Read the model definition and answer for the solid it produces. Units are mm, in the model's axes. A direction names the side the tool comes from. Coordinates: 2 decimals unless noted, no trailing zeros. Order: outer loops, then holes, each group sorted by start corner. A loop starts at its lowest first (then second) coordinate and runs counter-clockwise, first axis right, second up. Notation, with made-up numbers: (46, -19) - (102, -19) arc R25 ccw to (102, 2) - close; hole circle Ø4 at (73.25, -4.75). An arc over 180 degrees is marked (long way). Write item = value, one per line.
Autodesk Fusion 360 part; units mm, degrees
sketch "Sketch1" plane through (0, 0, 0) normal (1, 0, 0) x (0, 1, 0) in component "Doorknob_Revolve_Addition"
  line L0 (0, 0) -> (0, 31.75)
  line L1 (-25.4, 3.175) -> (-25.4, 16.51)
  line L2 (-31.75, 16.51) -> (-31.75, 27.94)
  line L3 (-31.75, 27.94) -> (-38.1, 27.94)
  line L4 (-38.1, 27.94) -> (-38.1, 39.37)
  line L5 (-25.4, 16.51) -> (-31.75, 16.51)
  line L6 (-38.1, 39.37) -> (-44.45, 39.37)
  line L7 (-44.45, 39.37) -> (-44.45, 50.8)
  line L8 (-44.45, 50.8) -> (-50.8, 50.8)
  line L9 (-50.8, 50.8) -> (-50.8, 39.37)
  line L10 (-50.8, 39.37) -> (-57.15, 39.37)
  line L11 (-57.15, 39.37) -> (-57.15, 27.94)
  line L12 (-57.15, 27.94) -> (-63.5, 27.94)
  line L13 (-63.5, 27.94) -> (-63.5, 16.51)
  line L14 (-63.5, 16.51) -> (-69.85, 16.51)
  line L15 (-69.85, 16.51) -> (-69.85, 6.35)
  line L16 (-76.2, 0) -> (0, 0)
  arc A0 (-69.85, 6.35) -> (-76.2, 0) centre (-69.85, 0) ccw
  line L17 (0, 31.75) -> (-3.175, 31.75)
  line L18 (-3.175, 31.75) -> (-3.175, 3.175)
  line L19 (-3.175, 3.175) -> (-25.4, 3.175)
  dimension "d4" = 76.2
  dimension "d5" = 31.75
  dimension "d6" = 50.8
  dimension "d10" = 11.43
  dimension "d11" = 11.43
  dimension "d12" = 11.43
  dimension "d13" = 6.35
  dimension "d14" = 6.35
  dimension "d15" = 6.35
  dimension "d16" = 6.35
  dimension "d20" = 6.35
  dimension "d22" = 3.175
  dimension "d23" = 3.175
  dimension "d24" = 22.225
revolve "Revolve1" add sketch "Sketch1" angle 360 about axis through (0, -76.2, 0) along (0, 1, 0) in component "Doorknob_Revolve_Addition"
component "Doorknob_Revolve_Addition" placed x (1, 0, 0) y (0, 1, 0) z (0, 0, 1) at (0, 0, 0)
equation "d5 = ( 2.5 / 2 ) * 1 in"
equation "d11 = d10"
equation "d12 = d10"
equation "d14 = d13"
equation "d15 = d14"
equation "d16 = d13"
1) Flat-ended cylindrical pins translate along their axes: pin 1 Ø6 at (x, z) = (-24.5, -33.5) entering from +Y; pin 2 Ø1.5 at (x, y) = (11, -37.5) entering from -Z; pin 3 Ø10 at (x, z) = (-5.5, -1) entering from -Y. Find the tip coordinate at first contact, or state that the pin passes through.
Returned:
pin_1 = -38.1
pin_2 = -37.93
pin_3 = -76.17
2) The part is cut by section D-D (x = 33.5). Determine the outline of the cut face in (y, z), and give its area (3 significant figures).
Returned:
outline = (-57.15, -20.68) - (-50.8, -20.68) - (-50.8, -38.19) - (-44.45, -38.19) - (-44.45, -20.68) - (-38.1, -20.68) - (-38.1, 20.68) - (-44.45, 20.68) - (-44.45, 38.19) - (-50.8, 38.19) - (-50.8, 20.68) - (-57.15, 20.68) - close
area = 1,010 mm^2
3) The part is cut by section C-C (z = -34.5). Determine the outline of the cut face in (x, y), and give its area (3 significant figures).
Returned:
outline = (-37.29, -50.8) - (-18.97, -50.8) - (-18.97, -57.15) - (18.97, -57.15) - (18.97, -50.8) - (37.29, -50.8) - (37.29, -44.45) - (18.97, -44.45) - (18.97, -38.1) - (-18.97, -38.1) - (-18.97, -44.45) - (-37.29, -44.45) - close
area = 955 mm^2
4) For faces 1 (the face through (23.96, -41.32, -31.24)), 2 (the face through (-12, -63.5, 12)), 3 (the face through (-12, -31.75, 12)), determine the directions among +Z, -Z, +X, -X, +Y, -Y from which every point of the face is accessible in a straight line to the end or side of a thin tool.
Returned:
face_1 = +Y
face_2 = -Y
face_3 = none
5) Determine the mould class of faces 4 (the face through (30.995, -1.61, -6.883)), 5 (the face through (0, 0, 0)), 6 (the face through (-4.959, -28.619, 15.748)) for opening direction Y: pulls with the +Y half, pulls with the -Y half, needs draft (parallel to the pull), parting line crosses it, or undercut.
Returned:
face_4 = needs draft
face_5 = pulls with the +Y half
face_6 = undercut
6) Straight lines are drawn through the part: line 1 along Y through (x, z) = (37, -10); line 2 along X through (y, z) = (-43, 1.5); line 3 along Y through (x, z) = (40.5, 10.5). For each, find the intervals that lie inside material, in ascending order. Write a range as from..to.
Returned:
line_1 = -57.15..-38.1
line_2 = -39.34..39.34
line_3 = -50.8..-44.45
